CAD build for the part. Positions are in the model's coordinates, mm. Face numbers are marked on the shaded views. Round coordinates to 2 decimals unless told otherwise and drop trailing zeros. Order: outer loops, then holes, each group sorted by start corner. A loop starts at its lowest first (then second) coordinate and runs counter-clockwise, first axis right, second up. Notation, with made-up numbers: M 16,48.5 L 25,48.5 A24 cw 25,71.5 Z; hole C 5.5,52 d5. An arc over 180 degrees is marked long. Answer as a JSON object with one key per item and string values. Group by question number.
Autodesk Inventor part; units mm, degrees
ref_plane "YZ Plane" through (0, 0, 0) normal (1, 0, 0) x (0, 1, 0)
ref_plane "XZ Plane" through (0, 0, 0) normal (0, 1, 0) x (-1, 0, 0)
ref_plane "XY Plane" through (0, 0, 0) normal (0, 0, 1) x (1, 0, 0)
sketch "Sketch1" plane through (0, 0, 0) normal (0, 0, 1) x (1, 0, 0)
  circle A0 centre (0, 0) radius 6.35
  dimension "d0" = 12.7
extrude "Extrusion1" add sketch "Sketch1" along normal blind 18
hole "Hole1" at (0, 0, 18) direction (0, 0, -1) diameter 5 end through all
fillet "Fillet1" radius 0.5 4 edges at (-6.35, 0, 18) (0, 2.5, 18) (0, 2.5, 0) (-6.35, 0, 0)
properties part number "Idler" material "Nylon-6/6"
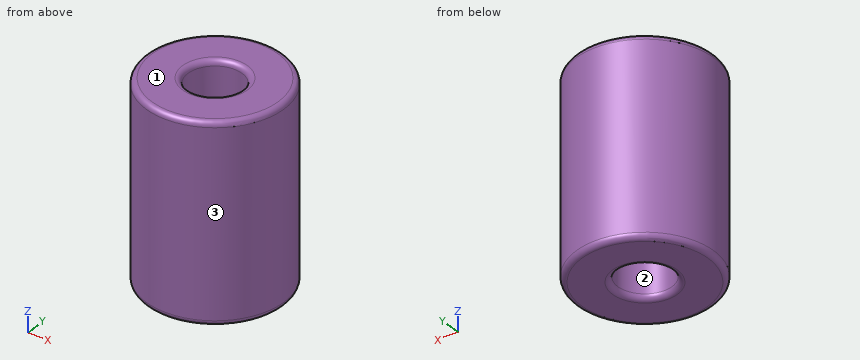
Item 1: Drill centre lines: line 1 (Y direction, x = 0, z = 9.5); line 2 (X direction, y = -0.75, z = 13); line 3 (X direction, y = -1.75, z = 10.75). Where is each one in solid material? Low to high. Write a range as [from, to].
Item 2: Cut at A-A, the plane x = 0. Give the cut face in (y, z), and give its area (3 significant figures).
Item 3: Two-plate mould, pull along X, no slides. Class the marked faces 1, 2 and 3: +X half, -X half, draft (parallel to the pull), parting line (faces both ways), or undercut.
Item 4: Flat gauge pins, fed straight in: pin 1 Ø3 at (x, y) = (-1.5, -4.5) entering from -Z; pin 2 Ø2 at (x, z) = (4, 4.5) entering from -Y. Where does each tip first touch, or does it go through?
Item 5: Cut at C-C, the plane z = 8.75. Give the cut face in (x, y), and give its area (3 significant figures).
Response values:
{
 "1": {"line 1": "[-6.35, -2.5], [2.5, 6.35]", "line 2": "[-6.31, -2.38], [2.38, 6.31]", "line 3": "[-6.1, -1.79], [1.79, 6.1]"},
 "2": {"outline": "M -6.35,0.5 A0.5 ccw -5.85,0 L -3,0 A0.5 ccw -2.5,0.5 L -2.5,17.5 A0.5 ccw -3,18 L -5.85,18 A0.5 ccw -6.35,17.5 Z; M 2.5,0.5 A0.5 ccw 3,0 L 5.85,0 A0.5 ccw 6.35,0.5 L 6.35,17.5 A0.5 ccw 5.85,18 L 3,18 A0.5 ccw 2.5,17.5 Z", "area": "138 mm^2"},
 "3": {"face 1": "draft", "face 2": "undercut", "face 3": "parting line"},
 "4": {"pin 1": "z = 0", "pin 2": "y = -5.6"},
 "5": {"outline": "C 0,0 d12.7; hole C 0,0 d5", "area": "107 mm^2"}
}
